from build123d import *

# Parameters (mm, degrees)
SKETCH1_W           = 47.5
SKETCH1_H           = 14
BOSS_EXTRUDE1_DEPTH = 6
BOSS_EXTRUDE2_DEPTH = 14
SKETCH4_R           = 4.1
CUT_EXTRUDE1_DEPTH  = 52.461150395
SKETCH5_R           = 1.65
CUT_EXTRUDE2_DEPTH  = 51.162236792
SKETCH6_R           = 3
CUT_EXTRUDE3_DEPTH  = 3
FILLET1_R           = 3
FILLET2_R           = 0.3


with BuildPart() as part:
    # Sketch1 → Boss-Extrude1 (new body)
    with BuildSketch(Plane(origin=(0, 0, 0), x_dir=(1, 0, 0), z_dir=(0, 1, 0))):
        with Locations((23.75, 7)):
            Rectangle(SKETCH1_W, SKETCH1_H)
    extrude(amount=BOSS_EXTRUDE1_DEPTH)

    # Sketch3 → Boss-Extrude2 (add)
    with BuildSketch(Plane.XY):
        with BuildLine():
            Line((15.75, 2.184089353), (16.718725156, 2.184089353))
            Line((16.718725156, 2.184089353), (30.781274844, 2.184089353))
            Line((30.781274844, 2.184089353), (31.75, 2.184089353))
            Line((31.75, 2.184089353), (31.75, 6))
            ThreePointArc((31.75, 6), (23.75, 14), (15.75, 6))
            Line((15.75, 6), (15.75, 2.184089353))
        make_face()
    extrude(amount=-BOSS_EXTRUDE2_DEPTH)

    # Sketch4 → Cut-Extrude1 (cut, through all)
    with BuildSketch(Plane.XY):
        with Locations((23.75, 6)):
            Circle(SKETCH4_R)
    extrude(amount=-CUT_EXTRUDE1_DEPTH, mode=Mode.SUBTRACT)

    # Sketch5 → Cut-Extrude2 (cut, through all)
    with BuildSketch(Plane(origin=(0, 6, 0), x_dir=(1, 0, 0), z_dir=(0, 1, 0))):
        with Locations(Location((5, 7, 0), (0, 0, 270))):
            Circle(SKETCH5_R)
        with Locations(Location((42.5, 7, 0), (0, 0, 90))):
            Circle(SKETCH5_R)
    extrude(amount=-CUT_EXTRUDE2_DEPTH, mode=Mode.SUBTRACT)

    # Sketch6 → Cut-Extrude3 (cut)
    with BuildSketch(Plane(origin=(0, 6, 0), x_dir=(1, 0, 0), z_dir=(0, 1, 0))):
        with Locations(Location((5, 7, 0), (0, 0, 270))):
            Circle(SKETCH6_R)
        with Locations(Location((42.5, 7, 0), (0, 0, 90))):
            Circle(SKETCH6_R)
    extrude(amount=-CUT_EXTRUDE3_DEPTH, mode=Mode.SUBTRACT)

    # Fillet1
    fillet1_edges = [part.edges().sort_by_distance(p)[0] for p in [
        (15.75, 6, -7),
        (31.75, 6, -7),
    ]]
    fillet(fillet1_edges, radius=FILLET1_R)

    # Fillet2
    fillet2_edges = [part.edges().sort_by_distance(p)[0] for p in [
        (47.5, 6, -7),
        (0, 6, -7),
        (47.5, 0, -7),
        (0, 0, -7),
    ]]
    fillet(fillet2_edges, radius=FILLET2_R)


solid = part.part
The model under review builds one solid part; all positions refer to its coordinate system, in mm. A direction names the side the tool comes from. Round coordinates to 2 decimals unless told otherwise and drop trailing zeros. Loops run counter-clockwise (first coordinate to the right, second up) from the corner with the lowest first, then second, coordinate; pieces in that order, holes last. Notation, with made-up numbers: M -36,48.25 L -13,48.25 A33 ccw -13,87.25 Z; hole C -1.5,-25.5 d5. An arc over 180 degrees is marked long. Answer as CSV lines item,"result". Start each with the question number.
Item 1: For faces 1 (the face through (8, 6, -9)), 2 (the face through (23, 0, -7)), 3 (the face through (39, 6, -7)), 4 (the face through (19.654, 6.18, -6.902)), 5 (the face through (3.85, 4.52, -4.23)), list the 3-axis set-ups (+Z, -Z, +X, -X, +Y, -Y) from which the entire face can be reached by the end or side of a thin tool; tool diameter is ignored.
Item 2: Consider section A-A (x = 5). Write out the cut boundary in (y, z), then the cut area to 3 significant figures.
Item 3: Consider section B-B (z = -12.25). Write out the cut boundary in (x, y).
Item 4: Consider section D-D (z = -7). State how many separate pieces and enclosed holes the cut face has, then the cut area to 3 significant figures.
Item 5: Insertion check: P1, Ø4, axis at x = 4.5, z = -6, coming from the +Y side; P2, Ø8, axis at x = 36, y = 6.5, coming from the +Z side; P3, Ø2, axis at x = 33.5, y = 11, coming from the -Z side; P4, Ø4, axis at x = 21.5, z = -10, coming from the +Y side. Each pin has a flat end and moves straight along its axis. Give the tip position at first contact, or say it passes through.
Item 6: Wall thickness on line 1 (X direction, y = 0.6, z = -7); line 2 (Z direction, x = 2.5, y = 5); line 3 (X direction, y = 3.9, z = -7): over which ranges is each line inside the solid? List them lowest first. Write a range as [from, to].
Item 7: Mouldability with a two-part tool opening along Z and no side actions: class faces 6 (the face through (23, 1, -14)), 7 (the face through (47.5, 3, -7)), 8 (the face through (3.7, 3, -5.7)) as released by +Z, released by -Z, zero draft, split by the parting line, or undercut.
Item 8: Consider section C-C (y = 4). Write out the cut boundary in (x, z).
Answer:
1,face 1,"+Z, -Z, -X, +Y"
1,face 2,"+Z, -Z, +X, -X, -Y"
1,face 3,"+Z, -Z, +X, +Y"
1,face 4,"+Z, -Z"
1,face 5,"+Y"
2,outline,"M 0,-14 L 6,-14 L 6,-10 L 3,-10 L 3,-8.65 L 0,-8.65 Z; M 0,-5.35 L 3,-5.35 L 3,-4 L 6,-4 L 6,0 L 0,0 Z"
2,area,"56.1 mm^2"
3,outline,"M 0,0.3 A0.3 ccw 0.3,0 L 47.2,0 A0.3 ccw 47.5,0.3 L 47.5,5.7 A0.3 ccw 47.2,6 L 34.33,6 A3 cw 31.45,8.18 A8 ccw 16.05,8.18 A3 cw 13.17,6 L 0.3,6 A0.3 ccw 0,5.7 Z; hole C 23.75,6 d8.2"
4,separate pieces,"3"
4,enclosed holes,"1"
4,area,"279 mm^2"
5,P1,"stops at y = 6"
5,P2,"stops at z = 0"
5,P3,"passes through"
5,P4,"stops at y = 14"
6,line 1,"x = [0, 3.35], [6.65, 40.85], [44.15, 47.5]"
6,line 2,"z = [-14, -8.66], [-5.34, 0]"
6,line 3,"x = [0, 2], [8, 20.23], [27.27, 39.5], [45.5, 47.5]"
7,face 6,"released by -Z"
7,face 7,"zero draft"
7,face 8,"undercut"
8,outline,"M 0,-14 L 20.17,-14 L 20.17,0 L 0,0 Z; M 27.33,-14 L 47.5,-14 L 47.5,0 L 27.33,0 Z; hole C 5,-7 d6; hole C 42.5,-7 d6"
